```python
from build123d import *

# Parameters (mm, degrees)
SKETCH_2_W          = 30
SKETCH_2_H          = 60
SKETCH_2_W_2        = 20
SKETCH_2_H_2        = 40
EXTRUDE_1_DEPTH     = 5
SKETCH_3_R          = 2
CUT_EXTRUDE_1_DEPTH = 5
EXTRUDE_2_DEPTH     = 5
SKETCH_6_R          = 1.5
CUT_EXTRUDE_2_DEPTH = 5
SKETCH_7_W          = 5
SKETCH_7_H          = 10
CUT_EXTRUDE_3_DEPTH = 100
SKETCH_8_W          = 30
SKETCH_8_H          = 5
EXTRUDE_3_DEPTH     = 80
SKETCH_9_W          = 30
SKETCH_9_H          = 5
EXTRUDE_4_DEPTH     = 60
SKETCH_11_W         = 30
SKETCH_11_H         = 8
EXTRUDE_5_DEPTH     = 32
EXTRUDE_6_DEPTH     = 30
SKETCH_14_W         = 30
SKETCH_14_H         = 5
EXTRUDE_7_DEPTH     = 30
SKETCH_15_W         = 37
SKETCH_15_H         = 100
EXTRUDE_8_DEPTH     = 30
SKETCH_12_R         = 3
CUT_EXTRUDE_5_DEPTH = 50
SKETCH_16_W         = 27
SKETCH_16_H         = 100
CUT_EXTRUDE_6_DEPTH = 30
SKETCH_17_R         = 3
CUT_EXTRUDE_7_DEPTH = 30
SKETCH_18_W         = 20
SKETCH_18_H         = 1
CUT_EXTRUDE_8_DEPTH = 10


with BuildPart() as part:
    # Sketch 2 → Extrude 1 (new body)
    with BuildSketch(Plane.XY):
        with Locations((10, -20)):
            Rectangle(SKETCH_2_W, SKETCH_2_H)
        with Locations((10, -20)):
            Rectangle(SKETCH_2_W_2, SKETCH_2_H_2, mode=Mode.SUBTRACT)
    extrude(amount=EXTRUDE_1_DEPTH)

    # Sketch 3 → Cut-Extrude 1 (cut)
    with BuildSketch(Plane.XY.offset(5)):
        with Locations((15.25, 5.5)):
            Circle(SKETCH_3_R)
        with Locations((15.25, -45.5)):
            Circle(SKETCH_3_R)
        with Locations((4.75, -45.5)):
            Circle(SKETCH_3_R)
        with Locations((4.75, 5.5)):
            Circle(SKETCH_3_R)
    extrude(amount=-CUT_EXTRUDE_1_DEPTH, mode=Mode.SUBTRACT)

    # Sketch 5 → Extrude 2 (add)
    with BuildSketch(Plane(origin=(25, 0, 0), x_dir=(0, 0, -1), z_dir=(1, 0, 0))):
        with BuildLine():
            Line((-5, -42), (-5, -40))
            Line((-5, -40), (0, -40))
            Line((0, -40), (0, -42))
            ThreePointArc((0, -42), (0.878679656, -44.121320344), (3, -45))
            Line((3, -45), (20, -45))
            Line((20, -45), (20, -50))
            Line((20, -50), (0, -50))
            Line((0, -50), (-5, -50))
            Line((-5, -50), (-25, -50))
            Line((-25, -50), (-25, -45))
            Line((-25, -45), (-8, -45))
            ThreePointArc((-8, -45), (-5.878679656, -44.121320344), (-5, -42))
        make_face()
    extrude_2 = extrude(amount=EXTRUDE_2_DEPTH)

    # Mirror 1: Extrude 2 across plane
    add(extrude_2.mirror(Plane(origin=(10, 0, 0), x_dir=(0, 0, 1), z_dir=(1, 0, 0))))

    # Sketch 6 → Cut-Extrude 2 (cut)
    with BuildSketch(Plane(origin=(0, -45, 0), x_dir=(1, 0, 0), z_dir=(0, 1, 0))):
        with Locations(Location((-7.5, 12.5, 0), (0, 0, 270))):
            Circle(SKETCH_6_R)
        with Locations(Location((-7.5, -17.5, 0), (0, 0, 270))):
            Circle(SKETCH_6_R)
        with Locations(Location((27.5, -17.5, 0), (0, 0, 270))):
            Circle(SKETCH_6_R)
        with Locations(Location((27.5, 12.5, 0), (0, 0, 270))):
            Circle(SKETCH_6_R)
    extrude(amount=-CUT_EXTRUDE_2_DEPTH, mode=Mode.SUBTRACT)

    # Sketch 7 → Cut-Extrude 3 (cut)
    with BuildSketch(Plane.XY.offset(25)):
        with Locations((27.5, -45)):
            Rectangle(SKETCH_7_W, SKETCH_7_H)
        with Locations((-7.5, -45)):
            Rectangle(SKETCH_7_W, SKETCH_7_H)
    extrude(amount=-CUT_EXTRUDE_3_DEPTH, mode=Mode.SUBTRACT)

    # Sketch 8 → Extrude 3 (add)
    with BuildSketch(Plane(origin=(0, 10, 0), x_dir=(1, 0, 0), z_dir=(0, 1, 0))):
        with Locations((10, -2.5)):
            Rectangle(SKETCH_8_W, SKETCH_8_H)
    extrude(amount=EXTRUDE_3_DEPTH)

    # Sketch 9 → Extrude 4 (add)
    with BuildSketch(Plane.XZ.offset(50)):
        with Locations((10, 2.5)):
            Rectangle(SKETCH_9_W, SKETCH_9_H)
    extrude(amount=EXTRUDE_4_DEPTH)

    # Sketch 11 → Extrude 5 (add)
    with BuildSketch(Plane.XY.offset(5)):
        with Locations((10, -106)):
            Rectangle(SKETCH_11_W, SKETCH_11_H)
        with Locations((10, 86)):
            Rectangle(SKETCH_11_W, SKETCH_11_H)
    extrude(amount=EXTRUDE_5_DEPTH)

    # Sketch 13 → Extrude 6 (add)
    with BuildSketch(Plane(origin=(0, -102, 0), x_dir=(1, 0, 0), z_dir=(0, 1, 0))):
        Polygon((-5, -37), (25, -37), (25, -34.408335309), (25, -32), (-5, -32), align=None)
    extrude(amount=EXTRUDE_6_DEPTH)

    # Sketch 14 → Extrude 7 (add)
    with BuildSketch(Plane.XZ.offset(-82)):
        with Locations((10, 34.5)):
            Rectangle(SKETCH_14_W, SKETCH_14_H)
    extrude(amount=EXTRUDE_7_DEPTH)

    # Sketch 15 → Extrude 8 (add)
    with BuildSketch(Plane.ZY.offset(5)):
        with Locations((18.5, -160)):
            Rectangle(SKETCH_15_W, SKETCH_15_H)
    extrude(amount=-EXTRUDE_8_DEPTH)

    # Sketch 12 → Cut-Extrude 5 (cut)
    with BuildSketch(Plane.XY.offset(5)):
        with Locations((0, 65)):
            Circle(SKETCH_12_R)
        with Locations((20, 65)):
            Circle(SKETCH_12_R)
    extrude(amount=CUT_EXTRUDE_5_DEPTH, mode=Mode.SUBTRACT)

    # Sketch 16 → Cut-Extrude 6 (cut)
    with BuildSketch(Plane(origin=(25, 0, 0), x_dir=(0, 0, -1), z_dir=(1, 0, 0))):
        with Locations((-18.5, -152)):
            Rectangle(SKETCH_16_W, SKETCH_16_H)
    extrude(amount=-CUT_EXTRUDE_6_DEPTH, mode=Mode.SUBTRACT)

    # Sketch 17 → Cut-Extrude 7 (cut)
    with BuildSketch(Plane.XY.offset(37)):
        with Locations((20, -190)):
            Circle(SKETCH_17_R)
        with Locations((0, -190)):
            Circle(SKETCH_17_R)
    extrude(amount=-CUT_EXTRUDE_7_DEPTH, mode=Mode.SUBTRACT)

    # Sketch 18 → Cut-Extrude 8 (cut)
    with BuildSketch(Plane(origin=(0, 0, 0), x_dir=(-1, 0, 0), z_dir=(0, 0, -1))):
        with Locations((-10, -40.5)):
            Rectangle(SKETCH_18_W, SKETCH_18_H)
        with Locations((-10, 0.5)):
            Rectangle(SKETCH_18_W, SKETCH_18_H)
    extrude(amount=-CUT_EXTRUDE_8_DEPTH, mode=Mode.SUBTRACT)


solid = part.part
```
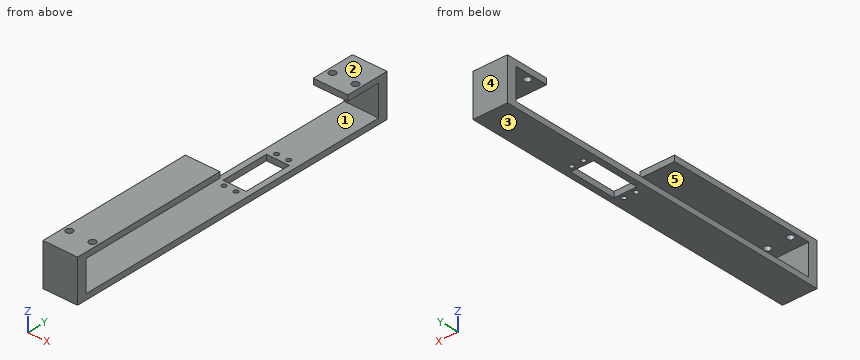
Model file for the job. Use its own axes, mm. Face numbers are marked on the shaded views. A direction names the side the tool comes from. Give positions to 0.01 mm unless a question says otherwise; leave off trailing zeros. Write each loop counter-clockwise with the first axis right and the second up, starting at its lowest first coordinate (ties: lowest second). Pieces come first, ordered by that corner, then holes. Notation, with made-up numbers: (5.5, 62) -> (30.5, 62) arc R25 ccw to (30.5, 83) -> close; hole circle Ø6 at (50.25, -3). An arc over 180 degrees is marked (long way). Use CSV: the item, a comma, the result in double quotes. Start each with the question number.
1) Cut at B-B on y = -110. List the corners of the cut face in (x, z).
2) Tool access for the marked faces 4 and 5: list every direction of +Z, -Z, +X, -X, +Y, -Y with a clear straight run to the whole face (end or side of a thin tool).
3) Drill centre lines: L1, parallel to Y at x = 4.75, z = 3.75; L2, parallel to X at y = -190, z = 35.6; L3, parallel to Y at x = 0, z = 35.1. Where is each one in solid material? Low to high.
4) Cut at A-A on z = 8. List the corners of the cut face in (x, y), plus the area to 3 significant figures.
5) Two-plate mould, pull along Z, no slides. Class the marked faces 1, 2 and 3: released by +Z, released by -Z, zero draft, split by the parting line, or undercut.
6) Pin check, flat tips, straight feed: P1, Ø3, axis at x = 15.25, y = 5.5, coming from the -Z side; P2, Ø12, axis at x = 0, y = -49, coming from the +Z side. Stop position of each tip, or through.
7) Cut at C-C on y = -190. List the corners of the cut face in (x, z).
Final values:
1,outline,"(-5, 0) -> (25, 0) -> (25, 5) -> (-5, 5) -> close; (-5, 32) -> (25, 32) -> (25, 37) -> (-5, 37) -> close"
2,face 4,"+Z, -Z, +X, -X, +Y"
2,face 5,"+X, -X"
3,L1,"y = -210 to -47.5, -43.5 to -41, 1 to 3.5, 7.5 to 90"
3,L2,"x = -5 to -3, 3 to 17, 23 to 25"
3,L3,"y = -210 to -193, -187 to -72, 52 to 62, 68 to 90"
4,outline,"(-5, -210) -> (25, -210) -> (25, -202) -> (-5, -202) -> close; (-5, 82) -> (25, 82) -> (25, 90) -> (-5, 90) -> close"
4,area,"480 mm2"
5,face 1,"undercut"
5,face 2,"released by +Z"
5,face 3,"released by -Z"
6,P1,"passes through"
6,P2,"stops at z = 5"
7,outline,"(-5, 0) -> (25, 0) -> (25, 5) -> (-5, 5) -> close; (-5, 32) -> (-3, 32) -> (-3, 37) -> (-5, 37) -> close; (3, 32) -> (17, 32) -> (17, 37) -> (3, 37) -> close; (23, 32) -> (25, 32) -> (25, 37) -> (23, 37) -> close"
